Check sheet for the drawn part. Datum: minimum x, y, z corner. Units: mm. A direction names the side the tool comes from. Round coordinates to 2 decimals unless told otherwise and drop trailing zeros. Write each loop counter-clockwise with the first axis right and the second up, starting at its lowest first coordinate (ties: lowest second). Pieces come first, ordered by that corner, then holes.
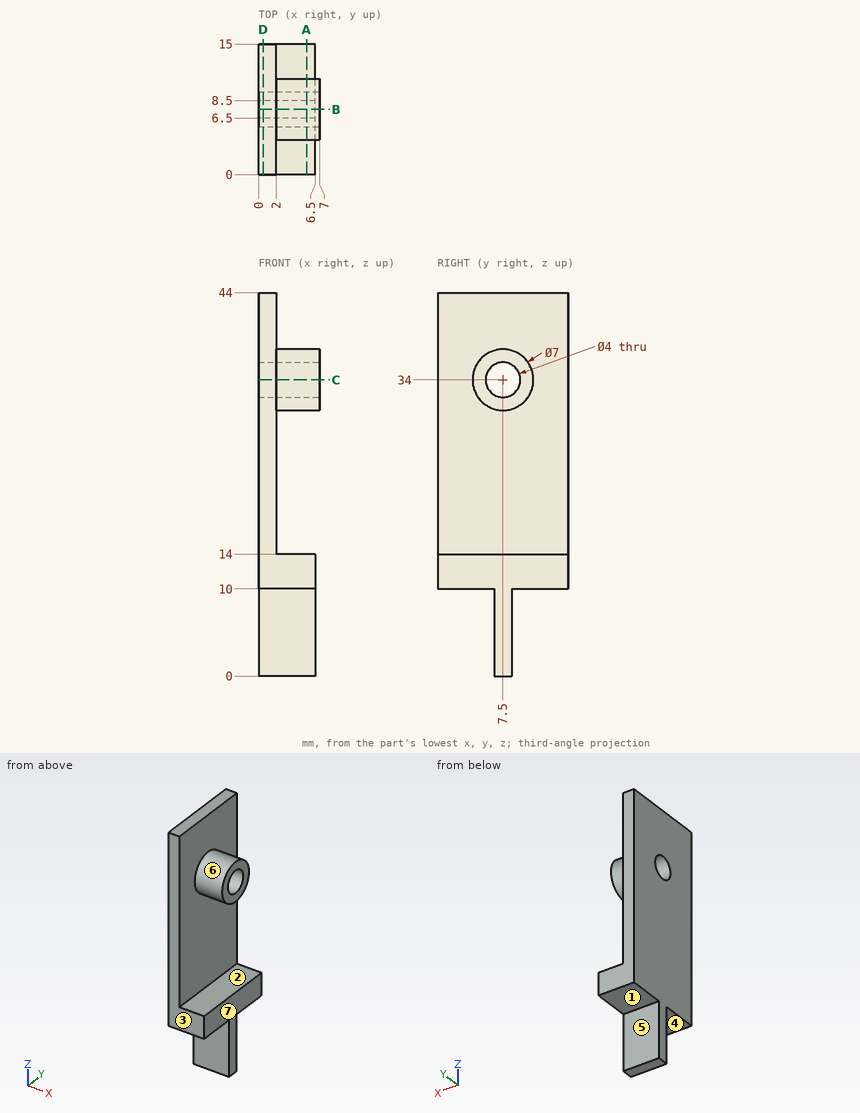
Q1. Material ranges on line 1 along Y through (x, z) = (4.25, 34); line 2 along Z through (x, y) = (6, 7.75); line 3 along Y through (x, z) = (1.75, 34), recorded low to high.
Recorded:
line 1: y = 4 to 5.5, 9.5 to 11
line 2: z = 0 to 14, 30.51 to 32.02, 35.98 to 37.49
line 3: y = 0 to 5.5, 9.5 to 15
Q2. Release check for a two-part mould opening along Z. For the marked faces 1, 2 and 3 record: released by +Z, released by -Z, zero draft, split by the parting line, or undercut.
Recorded:
face 1: released by -Z
face 2: undercut
face 3: zero draft
Q3. Sectioned sample at C-C (z = 34). Enter the section's corners in (x, y), plus the area to 3 significant figures.
Recorded:
outline: (0, 0) - (2, 0) - (2, 4) - (7, 4) - (7, 5.5) - (0, 5.5) - close; (0, 9.5) - (7, 9.5) - (7, 11) - (2, 11) - (2, 15) - (0, 15) - close
area: 37.0 mm2
Q4. Depth check by flat-ended pin: P1, Ø4.5, axis at y = 4.5, z = 30.5, coming from the +X side; P2, Ø4, axis at y = 6.5, z = 5, coming from the +X side; P3, Ø2, axis at x = 4.5, y = 4.5, coming from the -Z side; P4, Ø1.3, axis at x = 4, y = 10.5, coming from the +Z side. Enter the tip coordinate at first touch or a pass-through.
Recorded:
P1: stops at x = 7
P2: stops at x = 6.5
P3: stops at z = 10
P4: stops at z = 36.59
Q5. Sectioned sample at A-A (x = 5.5). Enter the section's corners in (y, z), plus the area to 3 significant figures.
Recorded:
outline: (0, 10) - (6.5, 10) - (6.5, 0) - (8.5, 0) - (8.5, 10) - (15, 10) - (15, 14) - (0, 14) - close; circle Ø7 at (7.5, 34); hole circle Ø4 at (7.5, 34)
area: 106 mm2
Q6. Tool access check on the marked faces 4, 5, 6 and 7. Record the directions out of +Z, -Z, +X, -X, +Y, -Y that give a thin tool (end or side, any length) a straight path to the whole face; none if there is none.
Recorded:
face 4: -Z, +X, -X, -Y
face 5: -Z, +X, -X, +Y
face 6: +X
face 7: -Z, +X, +Y, -Y
Q7. Sectioned sample at D-D (x = 0.5). Enter the section's corners in (y, z).
Recorded:
outline: (0, 10) - (6.5, 10) - (6.5, 0) - (8.5, 0) - (8.5, 10) - (15, 10) - (15, 44) - (0, 44) - close; hole circle Ø4 at (7.5, 34)
Q8. Sectioned sample at B-B (y = 7.5). Enter the section's corners in (x, z).
Recorded:
outline: (0, 0) - (6.5, 0) - (6.5, 14) - (2, 14) - (2, 30.5) - (7, 30.5) - (7, 32) - (0, 32) - close; (0, 36) - (7, 36) - (7, 37.5) - (2, 37.5) - (2, 44) - (0, 44) - close
